Source: CAD feature listing. Evaluate the final solid. Frame: model axes, mm. Face numbers are marked on the shaded views. Coordinates: 2 decimals unless noted, no trailing zeros. Loops run counter-clockwise (first coordinate to the right, second up) from the corner with the lowest first, then second, coordinate; pieces in that order, holes last. Notation, with made-up numbers: M -21,-18.75 L 28,-18.75 A15 cw 28,-10.75 Z; hole C 18.25,14 d7. An arc over 180 degrees is marked long. One line per question, with ' | ' between items. Start each with the question number.
1. Ray query, probe 1 along Z at (x, y) = (17, 1.1); probe 2 along Y at (x, z) = (0.5, -0.5). Return the intervals inside material, ascending.
2. Section query A-A, the plane y = 0.7. State how many separate pieces and enclosed holes the cut face has, and give its area (3 significant figures).
3. Mould query, pull axis X, two halves, no side actions, for the marked faces 1 and 2. Classes: pulls with the +X half, pulls with the -X half, needs draft (parallel to the pull), parting line crosses it, or undercut.
4. Section query B-B, the plane x = -4.5. Output: boundary loops of the cut face in (y, z), and give its area (3 significant figures).
5. Section query C-C, the plane z = 2.5. Output: boundary loops of the cut face in (x, y).
6. Pin query (flat end, axial travel): P1, Ø1, axis at x = -9.5, y = 1, coming from the -Z side; P2, Ø0.6, axis at y = 1, z = -2, coming from the +X side; P3, Ø0.6, axis at y = 1, z = -1.5, coming from the -X side. Return the tip coordinate at first contact, or that it passes through.
7. Section query D-D, the plane x = -12.5. Output: boundary loops of the cut face in (y, z), and give its area (3 significant figures).
```python
from build123d import *

# Parameters (mm, degrees)
SKETCH1_W           = 10
SKETCH1_H           = 0.6
BOSS_EXTRUDE1_DEPTH = 26.5
SKETCH2_W           = 5
SKETCH2_H           = 5
BOSS_EXTRUDE2_DEPTH = 1.2


with BuildPart() as part:
    # Sketch1 → Boss-Extrude1 (new, symmetric)
    with BuildSketch(Plane(origin=(0, 0, 0), x_dir=(0, 0, -1), z_dir=(1, 0, 0))):
        Rectangle(SKETCH1_W, SKETCH1_H)
    extrude(amount=BOSS_EXTRUDE1_DEPTH, both=True)

    # Sketch2 → Boss-Extrude2 (add)
    with BuildSketch(Plane(origin=(0, 0.3, 0), x_dir=(1, 0, 0), z_dir=(0, 1, 0))):
        with Locations((-15.714285714, 1.5)):
            Rectangle(SKETCH2_W, SKETCH2_H)
        with Locations((-22, 1.5)):
            Rectangle(SKETCH2_W, SKETCH2_H)
        with Locations((-9.428571429, 1.5)):
            Rectangle(SKETCH2_W, SKETCH2_H)
        with Locations((-3.142857143, 1.5)):
            Rectangle(SKETCH2_W, SKETCH2_H)
        with Locations((3.142857143, 1.5)):
            Rectangle(SKETCH2_W, SKETCH2_H)
        with Locations((9.428571429, 1.5)):
            Rectangle(SKETCH2_W, SKETCH2_H)
        with Locations((15.714285714, 1.5)):
            Rectangle(SKETCH2_W, SKETCH2_H)
        with Locations((22, 1.5)):
            Rectangle(SKETCH2_W, SKETCH2_H)
    extrude(amount=BOSS_EXTRUDE2_DEPTH)


solid = part.part
```
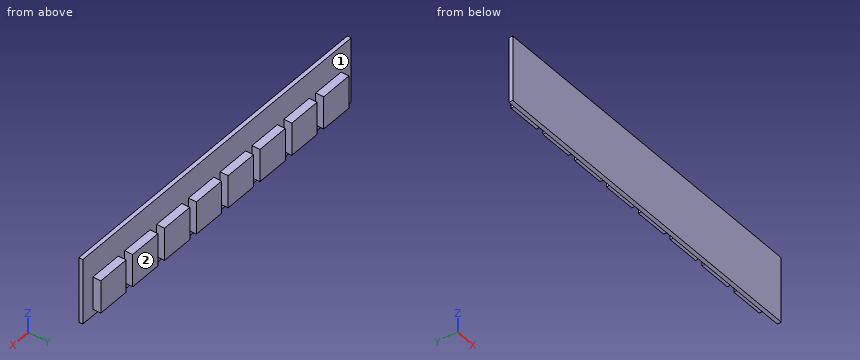
Taken from the geometry:
1) probe 1: -4 to 1 | probe 2: -0.3 to 0.3
2) separate pieces: 8 | enclosed holes: 0 | area: 200 mm^2
3) face 1: undercut | face 2: needs draft
4) outline: M -0.3,-5 L 0.3,-5 L 0.3,-4 L 1.5,-4 L 1.5,1 L 0.3,1 L 0.3,5 L -0.3,5 Z | area: 12.0 mm^2
5) outline: M -26.5,-0.3 L 26.5,-0.3 L 26.5,0.3 L -26.5,0.3 Z
6) P1: z = -4 | P2: x = 24.5 | P3: x = -24.5
7) outline: M -0.3,-5 L 0.3,-5 L 0.3,5 L -0.3,5 Z | area: 6.00 mm^2
